from build123d import *

# Parameters (mm, degrees)
SKETCH1_W           = 25.4
SKETCH1_H           = 6.35
BOSS_EXTRUDE1_DEPTH = 6.35


with BuildPart() as part:
    # Sketch1 → Boss-Extrude1 (new body)
    with BuildSketch(Plane(origin=(0, 0, 0), x_dir=(0, 0, -1), z_dir=(1, 0, 0))):
        Polygon((12.7, 215.9), (133.35, 215.9), (133.35, -215.9), (-133.35, -215.9), (-133.35, 215.9), (-12.7, 215.9), (-12.7, 209.55), (12.7, 209.55), align=None)
        with Locations((0, -187.325)):
            Rectangle(SKETCH1_W, SKETCH1_H, mode=Mode.SUBTRACT)
        with BuildLine():
            Line((-96.07, 94.458095238), (-96.07, -155.541904762))
            Line((-96.07, -155.541904762), (96.07, -155.541904762))
            Line((96.07, -155.541904762), (96.07, 94.458095238))
            ThreePointArc((96.07, 94.458095238), (0, 171.288491158), (-96.07, 94.458095238))
        make_face(mode=Mode.SUBTRACT)
    extrude(amount=BOSS_EXTRUDE1_DEPTH)


solid = part.part
The listing builds one solid part. Answer for the finished solid, in the listing's coordinates (mm). Give positions to 0.01 mm unless a question says otherwise; leave off trailing zeros. Order: outer loops, then holes, each group sorted by start corner. A loop starts at its lowest first (then second) coordinate and runs counter-clockwise, first axis right, second up. Notation, with made-up numbers: (28.25, -38) - (45.25, -38) arc R14 cw to (45.25, -20) - close; hole circle Ø8 at (45, 86.5). An arc over 180 degrees is marked (long way). Answer as CSV lines item,"result".
Q1. A cutting plane is placed at A-A, the plane y = -28.5. Determine the outline of the cut face in (x, z).
Answer key:
outline,"(0, -133.35) - (6.35, -133.35) - (6.35, -96.07) - (0, -96.07) - close; (0, 96.07) - (6.35, 96.07) - (6.35, 133.35) - (0, 133.35) - close"
Q2. Straight lines are drawn through the part: L1, parallel to Z at x = 4.25, y = -102.5; L2, parallel to Y at x = 3.25, z = 31; L3, parallel to Z at x = 6, y = -188. For each, find the intervals that lie inside material, in ascending order.
Answer key:
L1,"z = -133.35 to -96.07, 96.07 to 133.35"
L2,"y = -215.9 to -155.54, 166.28 to 215.9"
L3,"z = -133.35 to -12.7, 12.7 to 133.35"
Q3. A cutting plane is placed at B-B, the plane x = 1.75. Determine the outline of the cut face in (y, z), and give its area (3 significant figures).
Answer key:
outline,"(-215.9, -133.35) - (215.9, -133.35) - (215.9, -12.7) - (209.55, -12.7) - (209.55, 12.7) - (215.9, 12.7) - (215.9, 133.35) - (-215.9, 133.35) - close; hole (-190.5, -12.7) - (-184.15, -12.7) - (-184.15, 12.7) - (-190.5, 12.7) - close; hole (-155.54, -96.07) - (94.46, -96.07) arc R98.48 ccw to (94.46, 96.07) - (-155.54, 96.07) - close"
area,"55,800 mm^2"
Q4. Determine the mould class of faces 1 (the face through (0, 3, 117)), 2 (the face through (3.13, 171.27, -1.86)) for opening direction Y: pulls with the +Y half, pulls with the -Y half, needs draft (parallel to the pull), parting line crosses it, or undercut.
Answer key:
face 1,"needs draft"
face 2,"undercut"
Q5. This flat-tipped pin is pushed along its axis until it touches: pin 1 Ø1.5 at (x, z) = (2, 11.5) entering from +Y. Where does it stop, or does it pass through?
Answer key:
pin 1,"stops at y = 209.55"
Q6. A cutting plane is placed at C-C, the plane z = -25. Determine the outline of the cut face in (x, y), and give its area (3 significant figures).
Answer key:
outline,"(0, -215.9) - (6.35, -215.9) - (6.35, -155.54) - (0, -155.54) - close; (0, 168.06) - (6.35, 168.06) - (6.35, 215.9) - (0, 215.9) - close"
area,"687 mm^2"
